Input: part model. Units: mm. Frame: model coordinates. Face numbers are marked on the shaded views. A direction names the side the tool comes from. Round coordinates to 2 decimals unless told otherwise and drop trailing zeros. Loops run counter-clockwise (first coordinate to the right, second up) from the corner with the lowest first, then second, coordinate; pieces in that order, holes last. Notation, with made-up numbers: (-20, 47.5) - (-10, 47.5) arc R5 ccw to (-10, 52.5) - close; hole circle Ø5 at (-29, 1). An arc over 180 degrees is marked (long way). Use CSV: the item, a comma, the result in double quotes. Start each with the question number.
1. Pin query (flat end, axial travel): P1, Ø1, axis at x = 12.5, z = 0.5, coming from the -Y side; P2, Ø0.7, axis at y = -5.5, z = 3.5, coming from the -X side; P3, Ø5, axis at x = 11.5, y = 4, coming from the +Z side. Return the tip coordinate at first contact, or that it passes through.
2. Cut plane B-B (x = 10). Return loops of the section in (y, z).
3. Material intervals for probe 1 along X at (y, z) = (0.75, -4.25); probe 2 along Z at (x, y) = (6.5, -3); probe 3 along Z at (x, y) = (25, -3), sorted ascending. Write a range as from..to.
4. Cut plane A-A (x = 5.5). Return loops of the section in (y, z), and give its area (3 significant figures).
5. Pull-direction query (X, two-part tool) for the marked faces 3, 4 and 5; classes: +X half, -X half, draft (parallel to the pull), parting line (faces both ways), or undercut.
6. Access query for the marked faces 1 and 2. Directions: +Z, -Z, +X, -X, +Y, -Y. A direction counts if a zero-diameter tool reaches every point of the face in a straight line with its end or side. Return the directions, or none.
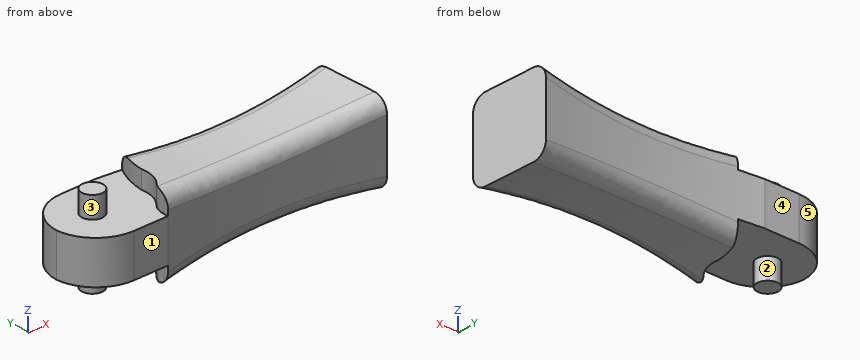
```python
from build123d import *

# Parameters (mm, degrees)
SKETCH1_W                = 6
SKETCH1_H                = 11.5
BOSS_EXTRUDE1_DEPTH      = 11
BOSS_EXTRUDE2_DEPTH      = 3
BOSS_EXTRUDE2_DEPTH_BACK = 9
SKETCH2_R                = 1.5
FILLET2_R                = 2
CUT_EXTRUDE4_DEPTH       = 3
FILLET8_R                = 3
CUT_EXTRUDE7_DEPTH       = 45.306461264
FILLET9_R                = 6


with BuildPart() as part:
    # Sketch1 → Boss-Extrude1 (new body)
    with BuildSketch(Plane(origin=(0, 0, 0), x_dir=(0, 0, -1), z_dir=(1, 0, 0))):
        Rectangle(SKETCH1_W, SKETCH1_H)
    extrude(amount=BOSS_EXTRUDE1_DEPTH)

    # Sketch2 → Boss-Extrude2 (add, two sides: drawn at the far end of the back side and taken through both)
    with BuildSketch(Plane.XY.offset(3).offset(-BOSS_EXTRUDE2_DEPTH_BACK)):
        with Locations((5.5, 0.25)):
            Circle(SKETCH2_R)
    extrude(amount=BOSS_EXTRUDE2_DEPTH + BOSS_EXTRUDE2_DEPTH_BACK)

    # Sketch3 → Loft1 section 0
    with BuildSketch(Plane(origin=(11, 0, 0), x_dir=(0, 0, -1), z_dir=(1, 0, 0))):
        with BuildLine():
            Line((5.75, -5.75), (-5.75, -5.75))
            Line((-5.75, -5.75), (-5.75, 5.75))
            Line((-5.75, 5.75), (5.75, 5.75))
            Line((5.75, 5.75), (5.75, -5.75))
        make_face()
    # Sketch4 → Loft1 section 1
    with BuildSketch(Plane(origin=(27, 0, 0), x_dir=(0, 0, -1), z_dir=(1, 0, 0))):
        with BuildLine():
            Line((4.75, -4.75), (-4.75, -4.75))
            Line((-4.75, -4.75), (-4.75, 4.75))
            Line((-4.75, 4.75), (4.75, 4.75))
            Line((4.75, 4.75), (4.75, -4.75))
        make_face()
    # Sketch5 → Loft1 section 2
    with BuildSketch(Plane(origin=(43, 0, 0), x_dir=(0, 0, -1), z_dir=(1, 0, 0))):
        with BuildLine():
            Line((5.75, -5.75), (-5.75, -5.75))
            Line((-5.75, -5.75), (-5.75, 5.75))
            Line((-5.75, 5.75), (5.75, 5.75))
            Line((5.75, 5.75), (5.75, -5.75))
        make_face()
    loft()

    # Fillet2
    fillet2_edges = [part.edges().sort_by_distance(p)[0] for p in [
        (27, 4.75, -4.75),
        (27, -4.75, -4.75),
        (27, -4.75, 4.75),
        (27, 4.75, 4.75),
    ]]
    fillet(fillet2_edges, radius=FILLET2_R)

    # Sketch11 → Cut-Extrude4 (cut)
    with BuildSketch(Plane(origin=(0, 0, -3), x_dir=(-1, 0, 0), z_dir=(0, 0, -1))):
        with BuildLine():
            Line((-8.5, 4.5), (-8.5, -4.5))
            ThreePointArc((-8.5, -4.5), (-13, 0), (-8.5, 4.5))
        make_face()
    cut_extrude4 = extrude(amount=CUT_EXTRUDE4_DEPTH, mode=Mode.SUBTRACT)

    # Mirror2: Cut-Extrude4 across plane
    add(cut_extrude4.mirror(Plane.XY), mode=Mode.SUBTRACT)

    # Fillet8
    fillet8_edges = [part.edges().sort_by_distance(p)[0] for p in [
        (11, 3.741657387, 4.375),
        (11, -3.741657387, 4.375),
        (11, 3.741657387, -4.375),
        (11, -3.741657387, -4.375),
    ]]
    fillet(fillet8_edges, radius=FILLET8_R)

    # Sketch14 → Cut-Extrude7 (cut, through all)
    with BuildSketch(Plane(origin=(0, 0, -3), x_dir=(-1, 0, 0), z_dir=(0, 0, -1))):
        with BuildLine():
            Line((-8.853025193, 6.183254842), (-15.095603268, 6.183254842))
            add(Edge.make_bspline(
                [(-12.96305568, 0.575442436), (-13.32215255, 3.608062735), (-15.095603268, 6.183254842)],
                knots=[0, 0, 0, 1, 1, 1], degree=2))
            Line((-12.96305568, 0.575442436), (-8.853025193, 6.183254842))
        make_face()
    cut_extrude7 = extrude(amount=CUT_EXTRUDE7_DEPTH, mode=Mode.SUBTRACT)

    # Mirror3: Cut-Extrude7 across plane
    add(cut_extrude7.mirror(Plane.XY), mode=Mode.SUBTRACT)

    # Fillet9
    # the kernel refuses this fillet: 6 mm, written as the material it takes off along each edge
    with BuildSketch(Plane(origin=(0, 5.75, 18), x_dir=(0, -1, 0), z_dir=(0, 0, -1))) as fillet9_piece_1:
        with BuildLine():
            CenterArc((FILLET9_R, -FILLET9_R), FILLET9_R, 90, 90)
            Line((0, -FILLET9_R), (0, 0))
            Line((0, 0), (FILLET9_R, 0))
        make_face()
    extrude(amount=36, mode=Mode.SUBTRACT)
    with BuildSketch(Plane(origin=(0, -5.75, -18), x_dir=(1, 0, 0), z_dir=(0, 0, 1))) as fillet9_piece_2:
        with BuildLine():
            CenterArc((FILLET9_R, FILLET9_R), FILLET9_R, 180, 90)
            Line((0, FILLET9_R), (0, 0))
            Line((0, 0), (FILLET9_R, 0))
        make_face()
    extrude(amount=36, mode=Mode.SUBTRACT)


solid = part.part
```
Established:
1,P1,"stops at y = -5.63"
1,P2,"stops at x = 11"
1,P3,"stops at z = 5.49"
2,outline,"(-5.75, -3) - (5.75, -3) - (5.75, 3) - (-5.75, 3) - close"
3,probe 1,"x = 4.09..6.91, 12.98..43"
3,probe 2,"z = -3..3"
3,probe 3,"z = -4.75..4.75"
4,outline,"(-5.73, -3) - (-1.25, -3) - (-1.25, -6) - (1.75, -6) - (1.75, -3) - (5.73, -3) - (5.73, 3) - (1.75, 3) - (1.75, 6) - (-1.25, 6) - (-1.25, 3) - (-5.73, 3) - close"
4,area,"86.7 mm2"
5,face 3,"undercut"
5,face 4,"draft"
5,face 5,"-X half"
6,face 1,"+Z, -Z, +X, -X, -Y"
6,face 2,"-Z"
